from build123d import *

# Parameters (mm, degrees)
SKETCH1_W           = 116.684502442
SKETCH1_H           = 63.5
SKETCH1_R           = 11
SKETCH1_R_2         = 2
SKETCH1_R_3         = 6
BOSS_EXTRUDE1_DEPTH = 6
CHAMFER1_SIZE       = 2.3
SKETCH2_R           = 6
SKETCH2_R_2         = 4.5
BOSS_EXTRUDE2_DEPTH = 2


with BuildPart() as part:
    # Sketch1 → Boss-Extrude1 (new body)
    with BuildSketch(Plane(origin=(0, 0, 0), x_dir=(1, 0, 0), z_dir=(0, 1, 0))):
        with Locations((26.592251221, 0)):
            Rectangle(SKETCH1_W, SKETCH1_H)
        Circle(SKETCH1_R, mode=Mode.SUBTRACT)
        with Locations((0, 21.5)):
            Circle(SKETCH1_R_2, mode=Mode.SUBTRACT)
        with Locations((18.619546181, -10.75)):
            Circle(SKETCH1_R_2, mode=Mode.SUBTRACT)
        with Locations((-18.619546181, -10.75)):
            Circle(SKETCH1_R_2, mode=Mode.SUBTRACT)
        with Locations((17.5, 0)):
            Circle(SKETCH1_R_3, mode=Mode.SUBTRACT)
        with Locations((-17.5, 0)):
            Circle(SKETCH1_R_3, mode=Mode.SUBTRACT)
    extrude(amount=BOSS_EXTRUDE1_DEPTH)

    # Chamfer1
    chamfer1_edges = [part.edges().sort_by_distance(p)[0] for p in [
        (-2, 6, -21.5),
        (16.619546181, 6, 10.75),
        (-20.619546181, 6, 10.75),
    ]]
    chamfer(chamfer1_edges, length=CHAMFER1_SIZE)

    # Sketch2 → Boss-Extrude2 (add)
    with BuildSketch(Plane.XZ):
        with Locations((-17.5, 0)):
            Circle(SKETCH2_R)
        with Locations((-17.5, 0)):
            Circle(SKETCH2_R_2, mode=Mode.SUBTRACT)
        with Locations((17.5, 0)):
            Circle(SKETCH2_R)
        with Locations((17.5, 0)):
            Circle(SKETCH2_R_2, mode=Mode.SUBTRACT)
    extrude(amount=-BOSS_EXTRUDE2_DEPTH)


solid = part.part
Build history of the part. All positions in model axes, mm. A direction names the side the tool comes from. Round coordinates to 2 decimals unless told otherwise and drop trailing zeros. Loops run counter-clockwise (first coordinate to the right, second up) from the corner with the lowest first, then second, coordinate; pieces in that order, holes last. Notation, with made-up numbers: (32.5, 86.25) -> (87.5, 86.25) arc R32 cw to (87.5, 125.25) -> close; hole circle Ø7 at (-12, 52). An arc over 180 degrees is marked (long way). One line per item, written item: value. Start each with the question number.
Q1. Two-plate mould, pull along Z, no slides. Class faces 3 (the face through (26, 3, 31.75)), 4 (the face through (84.935, 3, 0)), 5 (the face through (19.69, 1.82, 9.06)): released by +Z, released by -Z, zero draft, split by the parting line, or undercut.
Q2. Cut at A-A on z = 0. List the corners of the cut face in (x, y).
Q3. Probe line 1 along X through (y, z) = (4.95, 0); line 2 along X through (y, z) = (2.4, -21.5); line 3 along Z through (x, y) = (0, 1.1). List the from-to ranges inside material, lowest first.
Q4. 3-axis set-ups, long thin cutter, end or side, ignore diameter. For faces 1 (the face through (-22.26, 3.97, 3.65)), 2 (the face through (-22, 1, 0)): which of +Z, -Z, +X, -X, +Y, -Y reach the whole face in a straight line?
Q5. Cut at B-B on z = -9. List the corners of the cut face in (x, y).
Q6. Cut at C-C on x = 7.5. List the corners of the cut face in (y, z), plus the area to 3 significant figures.
Q7. Drop flat-ended pins along their axis: pin 1 Ø6.5 at (x, z) = (18.62, 10.75) entering from +Y; pin 2 Ø10.5 at (x, z) = (-17.5, 0) entering from +Y. Give the stop position or say it passes through.
Computed:
1. face 3: released by +Z
1. face 4: zero draft
1. face 5: undercut
2. outline: (-31.75, 0) -> (-22, 0) -> (-22, 2) -> (-23.5, 2) -> (-23.5, 6) -> (-31.75, 6) -> close; (-13, 0) -> (-11, 0) -> (-11, 6) -> (-11.5, 6) -> (-11.5, 2) -> (-13, 2) -> close; (11, 0) -> (13, 0) -> (13, 2) -> (11.5, 2) -> (11.5, 6) -> (11, 6) -> close; (22, 0) -> (84.93, 0) -> (84.93, 6) -> (23.5, 6) -> (23.5, 2) -> (22, 2) -> close
3. line 1: -31.75 to -23.5, -11.5 to -11, 11 to 11.5, 23.5 to 84.93
3. line 2: -31.75 to -2, 2 to 84.93
3. line 3: -31.75 to -23.5, -19.5 to -11, 11 to 31.75
4. face 1: +Y
4. face 2: +Y, -Y
5. outline: (-31.75, 0) -> (-6.32, 0) -> (-6.32, 6) -> (-31.75, 6) -> close; (6.32, 0) -> (84.93, 0) -> (84.93, 6) -> (6.32, 6) -> close
6. outline: (0, -31.75) -> (6, -31.75) -> (6, -8.05) -> (0, -8.05) -> close; (0, 8.05) -> (6, 8.05) -> (6, 31.75) -> (0, 31.75) -> close
6. area: 284 mm²
7. pin 1: y = 4.95
7. pin 2: y = 2
